```python
from build123d import *

# Parameters (mm, degrees)
SKETCH3_R           = 60
SKETCH3_R_2         = 40
BOSS_EXTRUDE1_DEPTH = 50
SKETCH4_R           = 60
SKETCH4_R_2         = 40
BOSS_EXTRUDE3_DEPTH = 50


with BuildPart() as part:
    # Sketch1 → Revolve1 (revolve)
    with BuildSketch(Plane.XY):
        Polygon((-70, -74.641016151), (-70, -500), (-60, -500), (-60, -75.957541127), (-40, -1.316524976), (-40, 2110), (-50, 2110), (-50, 0), align=None)
    revolve(axis=Axis((0, 0, 0), (0, 1, 0)))

    # Sketch3 → Boss-Extrude1 (add)
    with BuildSketch(Plane(origin=(0, 1860, 0), x_dir=(1, 0, 0), z_dir=(0, 1, 0))):
        Circle(SKETCH3_R)
        Circle(SKETCH3_R_2, mode=Mode.SUBTRACT)
    extrude(amount=BOSS_EXTRUDE1_DEPTH)

    # Sketch4 → Boss-Extrude3 (add)
    with BuildSketch(Plane(origin=(0, 600, 0), x_dir=(1, 0, 0), z_dir=(0, 1, 0))):
        Circle(SKETCH4_R)
        Circle(SKETCH4_R_2, mode=Mode.SUBTRACT)
    extrude(amount=-BOSS_EXTRUDE3_DEPTH)


solid = part.part
```
Source: CAD feature listing. Evaluate the final solid. Frame: model axes, mm. A direction names the side the tool comes from. Round coordinates to 2 decimals unless told otherwise and drop trailing zeros. Loops run counter-clockwise (first coordinate to the right, second up) from the corner with the lowest first, then second, coordinate; pieces in that order, holes last. Notation, with made-up numbers: M 71.5,21.5 L 98.5,21.5 A7 ccw 98.5,26.5 Z; hole C 32.25,43 d9. An arc over 180 degrees is marked long. Use a Markdown table: item, result. Add a question column.
1. Section query C-C on y = 356. Return the cut outline in (x, z).
2. Mould query, pull axis Z, two halves, no side actions, for faces 1 (the conical face through (-41.952, -21.528, -17.394)), 2 (the flat face through (-23, 1910, -45)), 3 (the cylindrical face through (55.55, -290.298, -42.594)). Classes: pulls with the +Z half, pulls with the -Z half, needs draft (parallel to the pull), parting line crosses it, or undercut.
3. Reachability of faces 4 (the flat face through (-22, 2110, 34)), 5 (the flat face through (-23, 1860, -45)), 6 (the cylindrical face through (59.94, -285.01, 2.64)), 7 (the cylindrical face through (-47.69, 2008.6, 15.02)), 8 (the flat face through (-52, -500, 31)) from +Z, -Z, +X, -X, +Y, -Y: full face, straight path, thin tool, end or side. Return the list, or none.
4. Contact query for flat-ended pins moving along their axis: P1, Ø12, axis at x = -26.5, y = 948, coming from the -Z side; P2, Ø6, axis at y = 382.5, z = -26, coming from the -X side; P3, Ø4, axis at x = 41, y = 1286.5, coming from the +Z side. Output: stop coordinate, or through.
5. Line query: line 1 (Z direction, x = 0, y = 1417); line 2 (Z direction, x = 0, y = -262.5); line 3 (X direction, y = 826.5, z = 5). Output: solid intervals per line, ascending.
Reported:
| question | item | result |
|---|---|---|
| 1 | outline | C 0,0 d100; hole C 0,0 d80 |
| 2 | face 1 | undercut |
| 2 | face 2 | needs draft |
| 2 | face 3 | parting line crosses it |
| 3 | face 4 | +Z, -Z, +X, -X, +Y |
| 3 | face 5 | none |
| 3 | face 6 | -Y |
| 3 | face 7 | +Y |
| 3 | face 8 | +Z, -Z, +X, -X, -Y |
| 4 | P1 | stops at z = -45.6 |
| 4 | P2 | stops at x = -44.4 |
| 4 | P3 | stops at z = 31.29 |
| 5 | line 1 | z = -50 to -40, 40 to 50 |
| 5 | line 2 | z = -70 to -60, 60 to 70 |
| 5 | line 3 | x = -49.75 to -39.69, 39.69 to 49.75 |
